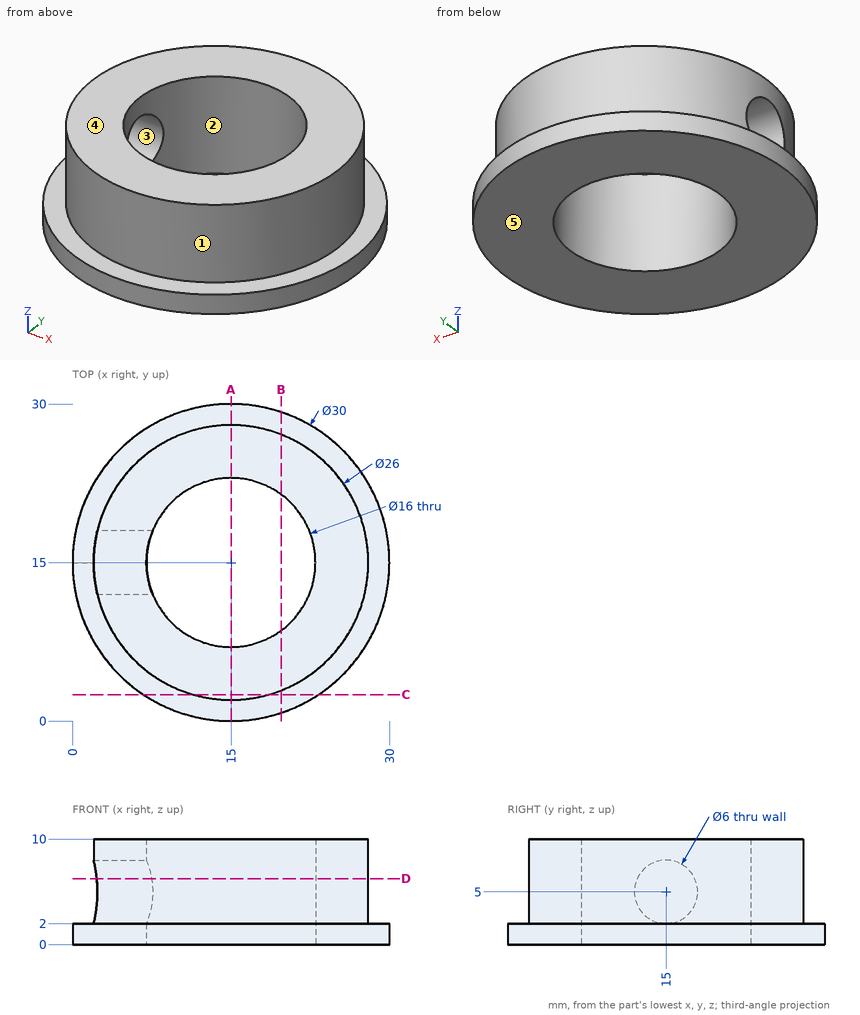
Part print with two shaded views. Sizes in mm from the minimum x, y, z corner. A direction names the side the tool comes from. Round coordinates to 2 decimals unless told otherwise and drop trailing zeros. Order: outer loops, then holes, each group sorted by start corner. A loop starts at its lowest first (then second) coordinate and runs counter-clockwise, first axis right, second up. Notation, with made-up numbers: (61.5, -23.75) - (87.5, -23.75) arc R21 cw to (87.5, -8.75) - close; hole circle Ø7 at (-28, 40.25). An arc over 180 degrees is marked (long way). Return JSON: item names as keys, results as strings.
(1) Pin check, flat tips, straight feed: pin 1 Ø6 at (x, y) = (3.5, 3.5) entering from +Z; pin 2 Ø1.5 at (x, y) = (21, 18.5) entering from +Z; pin 3 Ø1.5 at (y, z) = (8.5, 3.5) entering from +X; pin 4 Ø2 at (x, z) = (26.5, 2) entering from -Y. Stop position of each tip, or through.
Answer key:
{"pin 1": "stops at z = 2", "pin 2": "passes through", "pin 3": "stops at x = 26.66", "pin 4": "stops at y = 4.29"}
(2) Cut at B-B (x = 19.75). Give the cut face in (y, z).
Answer key:
{"outline": "(0.77, 0) - (8.56, 0) - (8.56, 10) - (2.9, 10) - (2.9, 2) - (0.77, 2) - close; (21.44, 0) - (29.23, 0) - (29.23, 2) - (27.1, 2) - (27.1, 10) - (21.44, 10) - close"}
(3) Tool access for the marked faces 1 and 2: list every direction of +Z, -Z, +X, -X, +Y, -Y with a clear straight run to the whole face (end or side of a thin tool).
Answer key:
{"face 1": "+Z", "face 2": "+Z, -Z"}
(4) Wall check: probe 1 along X at (y, z) = (15, 6.5); probe 2 along X at (y, z) = (8.5, 1.25); probe 3 along X at (y, z) = (11.5, 9). Give the ranges that are in metal, low to high. Write a range as from..to.
Answer key:
{"probe 1": "x = 23..28", "probe 2": "x = 1.48..10.34, 19.66..28.52", "probe 3": "x = 2.48..7.81, 22.19..27.52"}
(5) Cut at D-D (z = 6.25). Give the cut face in (x, y), then the cut area to 3 significant figures.
Answer key:
{"outline": "(2.29, 12.27) arc R13 ccw (long way) to (2.29, 17.73) - (7.48, 17.73) arc R8 cw (long way) to (7.48, 12.27) - close", "area": "302 mm^2"}
(6) Cut at C-C (y = 2.5). Give the cut face in (x, z).
Answer key:
{"outline": "(6.71, 0) - (23.29, 0) - (23.29, 2) - (18.57, 2) - (18.57, 10) - (11.43, 10) - (11.43, 2) - (6.71, 2) - close"}
(7) Cut at A-A (x = 15). Give the cut face in (y, z).
Answer key:
{"outline": "(0, 0) - (7, 0) - (7, 10) - (2, 10) - (2, 2) - (0, 2) - close; (23, 0) - (30, 0) - (30, 2) - (28, 2) - (28, 10) - (23, 10) - close"}
(8) Pull direction Z, two halves, no side cores. Call the marked faces 3, 4 and 5: +Z half, -Z half, draft (parallel to the pull), parting line (faces both ways), or undercut.
Answer key:
{"face 3": "undercut", "face 4": "+Z half", "face 5": "-Z half"}
